Input: part model. Units: mm. Frame: model coordinates. Give positions to 0.01 mm unless a question says otherwise; leave off trailing zeros. Answer as a JSON object with one key per item and string values. Group by question number.
(1) Pin query (flat end, axial travel): P1, Ø22, axis at x = 20.5, z = -21, coming from the +Y side; P2, Ø12, axis at x = 146, z = -27.5, coming from the +Y side; P3, Ø6, axis at x = 233, z = -29.5, coming from the +Y side; P4, Ø10, axis at x = 319.5, z = -32, coming from the +Y side. Return the tip coordinate at first contact, or that it passes through.
(2) Mould query, pull axis Z, two halves, no side actions, for faces 1 (the flat face through (592, 592, 0)), 2 (the flat face through (1200, 592, -592)), 3 (the conical face through (227.16, 1190.49, -20.16)). Classes: +Z half, -Z half, draft (parallel to the pull), parting line (faces both ways), or undercut.
(3) Material intervals for L1, parallel to X at y = 1146, z = -25; L2, parallel to X at y = 479, z = -25, sorted ascending.
```python
from build123d import *

# Parameters (mm, degrees)
SKETCH1_W           = 1200
SKETCH1_H           = 1200
BOSS_EXTRUDE1_DEPTH = 1200
SKETCH3_W           = 80
SKETCH3_H           = 30
CUT_EXTRUDE2_DEPTH  = 15
FILLET1_R           = 10
SKETCH4_R           = 10
CUT_EXTRUDE3_DEPTH  = 15
SKETCH5_R           = 10
CUT_EXTRUDE4_DEPTH  = 2070.8369501
SKETCH6_R           = 15
CUT_EXTRUDE5_DEPTH  = 100
SKETCH8_R           = 7.5
CUT_EXTRUDE6_DEPTH  = 100
SKETCH11_R          = 10
CUT_EXTRUDE7_DEPTH  = 250
CHAMFER1_SIZE       = 10
SKETCH12_R          = 10
CUT_EXTRUDE8_DEPTH  = 30.004
CHAMFER2_SIZE       = 10


with BuildPart() as part:
    # Sketch1 → Boss-Extrude1 (new body)
    with BuildSketch(Plane(origin=(0, 0, 0), x_dir=(1, 0, 0), z_dir=(0, 1, 0))):
        with Locations((600, 600)):
            Rectangle(SKETCH1_W, SKETCH1_H)
    extrude(amount=BOSS_EXTRUDE1_DEPTH)

    # Sketch3 → Cut-Extrude2 (cut)
    with BuildSketch(Plane(origin=(0, 1200, 0), x_dir=(1, 0, 0), z_dir=(0, 1, 0))):
        with Locations((50, 25)):
            Rectangle(SKETCH3_W, SKETCH3_H)
    extrude(amount=-CUT_EXTRUDE2_DEPTH, mode=Mode.SUBTRACT)

    # Fillet1
    fillet1_edges = [part.edges().sort_by_distance(p)[0] for p in [
        (10, 1192.5, -10),
        (10, 1192.5, -40),
        (90, 1192.5, -40),
        (90, 1192.5, -10),
    ]]
    fillet(fillet1_edges, radius=FILLET1_R)

    # Sketch4 → Cut-Extrude3 (cut)
    with BuildSketch(Plane(origin=(0, 1185, 0), x_dir=(1, 0, 0), z_dir=(0, 1, 0))):
        with Locations(Location((25, 25, 0), (0, 0, 270))):
            Circle(SKETCH4_R)
        with Locations(Location((75, 25, 0), (0, 0, 270))):
            Circle(SKETCH4_R)
    extrude(amount=-CUT_EXTRUDE3_DEPTH, mode=Mode.SUBTRACT)

    # Sketch5 → Cut-Extrude4 (cut, through all)
    with BuildSketch(Plane(origin=(0, 1185, 0), x_dir=(1, 0, 0), z_dir=(0, 1, 0))):
        with Locations(Location((50, 25, 0), (0, 0, 270))):
            Circle(SKETCH5_R)
    extrude(amount=-CUT_EXTRUDE4_DEPTH, mode=Mode.SUBTRACT)

    # Sketch6 → Cut-Extrude5 (cut)
    with BuildSketch(Plane(origin=(0, 1200, 0), x_dir=(1, 0, 0), z_dir=(0, 1, 0))):
        with Locations(Location((145.500055777, 25, 0), (0, 0, 270))):
            Circle(SKETCH6_R)
    extrude(amount=-CUT_EXTRUDE5_DEPTH, mode=Mode.SUBTRACT)

    # Sketch8 → Cut-Extrude6 (cut)
    with BuildSketch(Plane(origin=(0, 1100, 0), x_dir=(1, 0, 0), z_dir=(0, 1, 0))):
        with Locations(Location((145.500055777, 25, 0), (0, 0, 270))):
            Circle(SKETCH8_R)
    extrude(amount=-CUT_EXTRUDE6_DEPTH, mode=Mode.SUBTRACT)

    # Sketch11 → Cut-Extrude7 (cut)
    with BuildSketch(Plane(origin=(0, 1200, 0), x_dir=(1, 0, 0), z_dir=(0, 1, 0))):
        with Locations(Location((236.465344037, 25, 0), (0, 0, 270))):
            Circle(SKETCH11_R)
    extrude(amount=-CUT_EXTRUDE7_DEPTH, mode=Mode.SUBTRACT)

    # Chamfer1
    chamfer1_edges = [part.edges().sort_by_distance(p)[0] for p in [
        (236.465344037, 1200, -35),
    ]]
    chamfer(chamfer1_edges, length=CHAMFER1_SIZE)

    # Sketch12 → Cut-Extrude8 (cut)
    with BuildSketch(Plane(origin=(0, 1200, 0), x_dir=(1, 0, 0), z_dir=(0, 1, 0))):
        with Locations(Location((317.39806053, 31.612058329, 0), (0, 0, 270))):
            Circle(SKETCH12_R)
    extrude(amount=-CUT_EXTRUDE8_DEPTH, mode=Mode.SUBTRACT)

    # Chamfer2
    chamfer2_edges = [part.edges().sort_by_distance(p)[0] for p in [
        (317.39806053, 1200, -41.612058329),
    ]]
    chamfer(chamfer2_edges, length=CHAMFER2_SIZE)


solid = part.part
```
Recorded:
{
 "1": {"P1": "stops at y = 1200", "P2": "stops at y = 1100", "P3": "stops at y = 950", "P4": "stops at y = 1170"},
 "2": {"face 1": "+Z half", "face 2": "draft", "face 3": "undercut"},
 "3": {"L1": "x = 0 to 40, 60 to 130.5, 160.5 to 226.47, 246.47 to 1200", "L2": "x = 0 to 40, 60 to 1200"}
}
